Check sheet for the modelled part. Datum: model origin and axes. Units: mm. Give positions to 0.01 mm unless a question says otherwise; leave off trailing zeros. Order: outer loops, then holes, each group sorted by start corner. A loop starts at its lowest first (then second) coordinate and runs counter-clockwise, first axis right, second up. Notation, with made-up numbers: (31, 10.25) -> (70, 10.25) arc R25 ccw to (70, 44.25) -> close; hole circle Ø2 at (49.25, 32). An arc over 180 degrees is marked (long way). Answer in a Markdown table with one row per item. Add a question column.
(1) Release check for a two-part mould opening along Z. For faces 1 (the face through (-7.705, 2.972, 3.955)), 2 (the face through (-1.08, 2.46, -4.88)), 3 (the face through (-7.277, 2.972, -4.695)) record: released by +Z, released by -Z, zero draft, split by the parting line, or undercut.
(2) Cross-section at D-D (z = -7). Record the cut outline in (x, y), then the cut area to 3 significant figures.
(3) Go/stop test with flat-tipped pins: pin 1 (1.5 mm diameter, centred on y = 2, z = 0.5, fed in from -X); pin 2 (3 mm diameter, centred on y = 4, z = -5, fed in from -X). Record where each tip stops, or that it passes through.
(4) Cross-section at C-C (z = 1). Record the cut outline in (x, y), then the cut area to 3 significant figures.
(5) Cross-section at A-A (y = 3.2). Record the cut outline in (x, z), then the cut area to 3 significant figures.
(6) Thickness scan on L1, parallel to Y at x = 6.5, z = -5; L2, parallel to X at y = 1.5, z = 0; L3, parallel to X at y = 0.6, z = -1. Record the ranges inside material, lowest first. Write a range as [from, to].
(7) Cross-section at B-B (x = -3.5). Record the cut outline in (y, z), then the cut area to 3 significant figures.
Autodesk Fusion 360 part; units mm, degrees
sketch "Sketch1" plane through (0, 0, 0) normal (0, 1, 0) x (1, 0, 0)
  circle A0 centre (0, 0) radius 5
  line L0 (4.6379, -8.8595) -> (9.9915, -0.4132)
  line L1 (9.9915, -0.4132) -> (5.3536, 8.4463)
  line L2 (5.3536, 8.4463) -> (-4.6379, 8.8595)
  line L3 (-4.6379, 8.8595) -> (-9.9915, 0.4132)
  line L4 (-9.9915, 0.4132) -> (-5.3536, -8.4463)
  line L5 (-5.3536, -8.4463) -> (4.6379, -8.8595)
  dimension "d1" = 10
extrude "Extrude1" add sketch "Sketch1" along normal blind 5
chamfer "Chamfer1" distance 1 angle 45 6 edges at (-7.3147, 0, -4.6363) (-7.6725, 0, 4.0165) (-0.3578, 0, 8.6529) (7.3147, 0, 4.6363) (7.6725, 0, -4.0165) (0.3578, 0, -8.6529)
thread "Thread1"
Answer below:
| question | item | result |
|---|---|---|
| 1 | face 1 | released by +Z |
| 1 | face 2 | undercut |
| 1 | face 3 | released by -Z |
| 2 | outline | (-5.82, 1) -> (-4.63, 0) -> (4.98, 0) -> (6.11, 1) -> (6.11, 5) -> (-5.82, 5) -> close |
| 2 | area | 58.5 mm² |
| 3 | pin 1 | stops at x = -9.91 |
| 3 | pin 2 | stops at x = -8.03 |
| 4 | outline | (-9.25, 1) -> (-8.12, 0) -> (-4.9, 0) -> (-4.9, 5) -> (-9.25, 5) -> close; (4.9, 0) -> (8.44, 0) -> (9.62, 1) -> (9.62, 5) -> (4.9, 5) -> close |
| 4 | area | 44.2 mm² |
| 5 | outline | (-9.99, -0.41) -> (-4.64, -8.86) -> (5.35, -8.45) -> (9.99, 0.41) -> (4.64, 8.86) -> (-5.35, 8.45) -> close; hole circle Ø10 at (0, 0) |
| 5 | area | 181 mm² |
| 6 | L1 | y = [0.42, 5] |
| 6 | L2 | x = [-9.78, -5], [5, 9.78] |
| 6 | L3 | x = [-9.15, -4.9], [4.9, 8.8] |
| 7 | outline | (0, -7.81) -> (1, -8.81) -> (5, -8.81) -> (5, -3.57) -> (0, -3.57) -> close; (0, 3.57) -> (5, 3.57) -> (5, 8.52) -> (1, 8.52) -> (0, 7.52) -> close |
| 7 | area | 50.0 mm² |
